```python
from build123d import *

# Parameters (mm, degrees)
SKETCH1_W             = 150
SKETCH1_H             = 110
BOSS_EXTRUDE2_DEPTH   = 10
SKETCH2_R             = 22.49
CUT_EXTRUDE1_DEPTH    = 6
F_5_0MM_DOWEL_HOLE1_D = 5
F_5_0MM_DOWEL_HOLE2_D = 5


with BuildPart() as part:
    # Sketch1 → Boss-Extrude2 (new body)
    with BuildSketch(Plane.XY):
        with Locations((-50.323383085, -0.820895522)):
            Rectangle(SKETCH1_W, SKETCH1_H)
    extrude(amount=BOSS_EXTRUDE2_DEPTH)

    # Sketch2 → Cut-Extrude1 (cut)
    with BuildSketch(Plane.XY.offset(10)):
        with Locations((-50.323383085, 0)):
            Circle(SKETCH2_R)
    extrude(amount=-CUT_EXTRUDE1_DEPTH, mode=Mode.SUBTRACT)

    # Ø5.0mm Dowel Hole1 (through all)
    with Locations(Plane(origin=(-50.323383085, 17.5, 4), x_dir=(1, 0, 0), z_dir=(0, 0, 1))):
        with Locations((0, 0), (-12.37436867, -5.125631329), (-17.5, -17.5), (-12.37436867, -29.874368671), (0, -35), (12.374368671, -29.874368671), (17.5, -17.5), (12.374368671, -5.125631329)):
            Hole(F_5_0MM_DOWEL_HOLE1_D / 2)

    # Ø5.0mm Dowel Hole2 (through all)
    with Locations(Plane(origin=(-110.323383085, 34.179104478, 10), x_dir=(1, 0, 0), z_dir=(0, 0, 1))):
        with Locations((0, 0), (125, 0), (125, -70), (0, -70)):
            Hole(F_5_0MM_DOWEL_HOLE2_D / 2)


solid = part.part
```
Work out the finished part from the listing and answer in its coordinate system (mm). A direction names the side the tool comes from. Round coordinates to 2 decimals unless told otherwise and drop trailing zeros. Write each loop counter-clockwise with the first axis right and the second up, starting at its lowest first coordinate (ties: lowest second). Pieces come first, ordered by that corner, then holes.
1) A cutting plane is placed at B-B on z = 5.5. Determine the outline of the cut face in (x, y).
2) Which of the six approach directions +Z, -Z, +X, -X, +Y, -Y give full straight-line access (tool end or side, diameter ignored) to faces 4 (the face through (-51, 24, 10)), 5 (the face through (-51, 0, 4))?
3) A cutting plane is placed at C-C on y = -17.5. Determine the outline of the cut face in (x, z).
4) A flat-ended cylindrical pin translates along its axis: P1, Ø8, axis at x = -62.7, y = 12.37, coming from the +Z side. Find the tip coordinate at first contact, or state that the pin passes through.
5) Consider probe 1 along X at (y, z) = (33, 5.25); probe 2 along X at (y, z) = (32, 5.5); probe 3 along Y at (x, z) = (16, 6.25). Determine where each line is inside the solid, lowest interval first.
6) A cutting plane is placed at A-A on y = 0. Determine the outline of the cut face in (x, z), and give its area (3 significant figures).
7) Determine the mould class of faces 1 (the face through (24.677, -2, 5)), 2 (the face through (-51, 54.179, 5)), 3 (the face through (-70.21, 0.75, 1.97)) for opening direction X: pulls with the +X half, pulls with the -X half, needs draft (parallel to the pull), parting line crosses it, or undercut.
Entries:
1. outline: (-125.32, -55.82) - (24.68, -55.82) - (24.68, 54.18) - (-125.32, 54.18) - close; hole circle Ø5 at (-110.32, -35.82); hole circle Ø5 at (-110.32, 34.18); hole circle Ø44.98 at (-50.32, 0); hole circle Ø5 at (14.68, -35.82); hole circle Ø5 at (14.68, 34.18)
2. face 4: +Z, +X, -X, +Y, -Y
2. face 5: +Z
3. outline: (-125.32, 0) - (-52.82, 0) - (-52.82, 4) - (-64.45, 4) - (-64.45, 10) - (-125.32, 10) - close; (-47.82, 0) - (24.68, 0) - (24.68, 10) - (-36.2, 10) - (-36.2, 4) - (-47.82, 4) - close
4. P1: stops at z = 4
5. probe 1: x = -125.32 to -112.53, -108.12 to 12.47, 16.88 to 24.68
5. probe 2: x = -125.32 to -111.55, -109.1 to 13.45, 15.9 to 24.68
5. probe 3: y = -55.82 to -37.94, -33.7 to 32.06, 36.3 to 54.18
6. outline: (-125.32, 0) - (-70.32, 0) - (-70.32, 4) - (-72.81, 4) - (-72.81, 10) - (-125.32, 10) - close; (-65.32, 0) - (-35.32, 0) - (-35.32, 4) - (-65.32, 4) - close; (-30.32, 0) - (24.68, 0) - (24.68, 10) - (-27.83, 10) - (-27.83, 4) - (-30.32, 4) - close
6. area: 1,190 mm2
7. face 1: pulls with the +X half
7. face 2: needs draft
7. face 3: undercut
